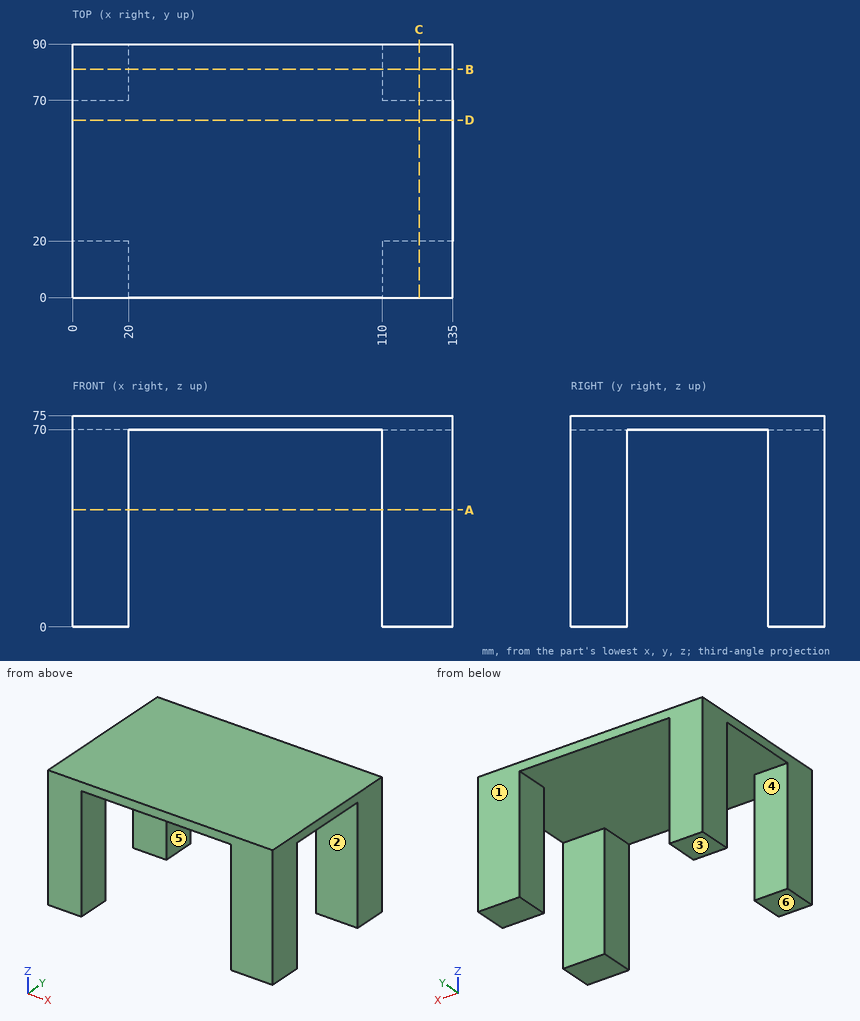
Check sheet for the drawn part. Datum: minimum x, y, z corner. Units: mm. A direction names the side the tool comes from. Round coordinates to 2 decimals unless told otherwise and drop trailing zeros. Write each loop counter-clockwise with the first axis right and the second up, starting at its lowest first coordinate (ties: lowest second). Pieces come first, ordered by that corner, then holes. Notation, with made-up numbers: (42, 67) - (50, 67) arc R28 ccw to (50, 96) - close; hole circle Ø2 at (67.25, -35.75). An arc over 180 degrees is marked (long way). Return JSON: item names as keys, results as strings.
Q1. Depth check by flat-ended pin: P1, Ø5, axis at x = 48.5, y = 43, coming from the -Z side; P2, Ø22, axis at y = 6, z = 25.5, coming from the -X side. Enter the tip coordinate at first touch or a pass-through.
Returned:
{"P1": "stops at z = 70", "P2": "stops at x = 0"}
Q2. Scan lines: L1, parallel to Y at x = 9, z = 24.5; L2, parallel to X at y = 10.5, z = 37; L3, parallel to Z at x = 61.5, y = 50.5. Record each from-to range of solid material in increasing order. Write a range as from..to.
Returned:
{"L1": "y = 0..20, 70..90", "L2": "x = 0..20, 110..135", "L3": "z = 70..75"}
Q3. Access from +Z, -Z, +X, -X, +Y, -Y to the whole of each face (thin tool, end or side, straight path). Record for the marked faces 4, 5 and 6.
Returned:
{"face 4": "-Z, +X, -X", "face 5": "-Z, +Y, -Y", "face 6": "-Z, +X, -X, +Y, -Y"}
Q4. Cross-section at C-C (x = 123). Record the boundary of the cut face in (y, z).
Returned:
{"outline": "(0, 0) - (20, 0) - (20, 70) - (70, 70) - (70, 0) - (90, 0) - (90, 75) - (0, 75) - close"}
Q5. Cross-section at A-A (z = 41.5). Record the boundary of the cut face in (x, y), then the cut area to 3 significant figures.
Returned:
{"outline": "(0, 0) - (20, 0) - (20, 20) - (0, 20) - close; (0, 70) - (20, 70) - (20, 90) - (0, 90) - close; (110, 0) - (135, 0) - (135, 20) - (110, 20) - close; (110, 70) - (135, 70) - (135, 90) - (110, 90) - close", "area": "1,800 mm²"}
Q6. Cross-section at B-B (y = 81). Record the boundary of the cut face in (x, z), then the cut area to 4 significant figures.
Returned:
{"outline": "(0, 0) - (20, 0) - (20, 70) - (110, 70) - (110, 0) - (135, 0) - (135, 75) - (0, 75) - close", "area": "3,825 mm²"}
Q7. Cross-section at D-D (y = 63). Record the boundary of the cut face in (x, z), then the cut area to 3 significant figures.
Returned:
{"outline": "(0, 70) - (135, 70) - (135, 75) - (0, 75) - close", "area": "675 mm²"}
Q8. Draft check along Y on the marked faces 1, 2 and 3. Enter one of: released by +Y, released by -Y, zero draft, split by the parting line, or undercut.
Returned:
{"face 1": "released by +Y", "face 2": "undercut", "face 3": "zero draft"}
